```python
from build123d import *

# Parameters (mm, degrees)
SKETCH_1_W          = 1980
SKETCH_1_H          = 530
SKETCH_1_W_2        = 1920
SKETCH_1_H_2        = 470
EXTRUDE_1_DEPTH     = 30
SKETCH_2_W          = 68
SKETCH_2_H          = 30
EXTRUDE_2_DEPTH     = 68
SKETCH_3_R          = 23.5
CUT_EXTRUDE_1_DEPTH = 1125.999555555
SKETCH_4_W          = 31
SKETCH_4_H          = 470
EXTRUDE_3_DEPTH     = 30
SKETCH_5_R          = 3
CUT_EXTRUDE_2_DEPTH = 1030.528532873
SKETCH_6_R          = 3
CUT_EXTRUDE_3_DEPTH = 1030.528532873
SKETCH_7_W          = 917.525313644
SKETCH_7_H          = 30
CUT_EXTRUDE_4_DEPTH = 1125.999555555
SKETCH_8_R          = 3
CUT_EXTRUDE_5_DEPTH = 1125.999555555
SKETCH_9_R          = 3
CUT_EXTRUDE_6_DEPTH = 1028.107102497
SKETCH_10_R         = 3
CUT_EXTRUDE_7_DEPTH = 1125.999555555


with BuildPart() as part:
    # 草图1 → 凸台-拉伸1 (new body)
    with BuildSketch(Plane(origin=(0, 0, 0), x_dir=(1, 0, 0), z_dir=(0, 1, 0))):
        Rectangle(SKETCH_1_W, SKETCH_1_H)
        Rectangle(SKETCH_1_W_2, SKETCH_1_H_2, mode=Mode.SUBTRACT)
    extrude(amount=EXTRUDE_1_DEPTH)

    # 草图2 → 凸台-拉伸2 (add)
    with BuildSketch(Plane.XZ):
        with Locations((0, 250)):
            Rectangle(SKETCH_2_W, SKETCH_2_H)
        with Locations((0, -250)):
            Rectangle(SKETCH_2_W, SKETCH_2_H)
    extrude(amount=EXTRUDE_2_DEPTH)

    # 草图3 → 切除-拉伸1 (cut, through all)
    with BuildSketch(Plane.XY.offset(265)):
        with Locations((0, -30)):
            Circle(SKETCH_3_R)
    extrude(amount=-CUT_EXTRUDE_1_DEPTH, mode=Mode.SUBTRACT)

    # 草图4 → 凸台-拉伸3 (add)
    with BuildSketch(Plane(origin=(0, 30, 0), x_dir=(1, 0, 0), z_dir=(0, 1, 0))):
        with Locations((764.5, 0)):
            Rectangle(SKETCH_4_W, SKETCH_4_H)
    extrude(amount=-EXTRUDE_3_DEPTH)

    # 草图5 → 切除-拉伸2 (cut, through all)
    with BuildSketch(Plane(origin=(0, 30, 0), x_dir=(1, 0, 0), z_dir=(0, 1, 0))):
        with Locations(Location((757, 180, 0), (0, 0, 270))):
            Circle(SKETCH_5_R)
        with Locations(Location((772.5, 180, 0), (0, 0, 270))):
            Circle(SKETCH_5_R)
        with Locations(Location((757, -180, 0), (0, 0, 270))):
            Circle(SKETCH_5_R)
        with Locations(Location((772.5, -180, 0), (0, 0, 270))):
            Circle(SKETCH_5_R)
    extrude(amount=-CUT_EXTRUDE_2_DEPTH, mode=Mode.SUBTRACT)

    # 草图6 → 切除-拉伸3 (cut, symmetric)
    with BuildSketch(Plane(origin=(0, 30, 0), x_dir=(1, 0, 0), z_dir=(0, 1, 0))):
        with Locations(Location((840, -250, 0), (0, 0, 270))):
            Circle(SKETCH_6_R)
    cut_extrude_3 = extrude(amount=CUT_EXTRUDE_3_DEPTH, both=True, mode=Mode.SUBTRACT)

    # 镜向1: 切除-拉伸3 across plane
    add(cut_extrude_3.mirror(Plane.XY), mode=Mode.SUBTRACT)

    # 草图7 → 切除-拉伸4 (cut, through all)
    with BuildSketch(Plane.XY.offset(265)):
        with Locations((-608.762656822, 15)):
            Rectangle(SKETCH_7_W, SKETCH_7_H)
    extrude(amount=-CUT_EXTRUDE_4_DEPTH, mode=Mode.SUBTRACT)

    # 草图8 → 切除-拉伸5 (cut, through all)
    with BuildSketch(Plane.XY.offset(265)):
        with Locations((-100, 15)):
            Circle(SKETCH_8_R)
    extrude(amount=-CUT_EXTRUDE_5_DEPTH, mode=Mode.SUBTRACT)

    # 草图9 → 切除-拉伸6 (cut, through all)
    with BuildSketch(Plane.XZ):
        with Locations(Location((110, 250, 0), (0, 0, 270))):
            Circle(SKETCH_9_R)
        with Locations(Location((44, 250, 0), (0, 0, 270))):
            Circle(SKETCH_9_R)
    cut_extrude_6 = extrude(amount=-CUT_EXTRUDE_6_DEPTH, mode=Mode.SUBTRACT)

    # 镜向2: 切除-拉伸6 across plane
    add(cut_extrude_6.mirror(Plane.XY), mode=Mode.SUBTRACT)

    # 草图10 → 切除-拉伸7 (cut, through all)
    with BuildSketch(Plane.XY.offset(265)):
        with Locations((-135, 15)):
            Circle(SKETCH_10_R)
    extrude(amount=-CUT_EXTRUDE_7_DEPTH, mode=Mode.SUBTRACT)


solid = part.part
```
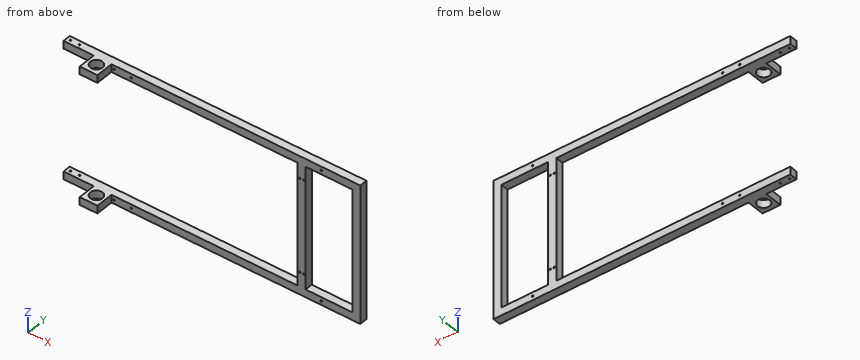
Check sheet for the modelled part. Datum: model origin and axes. Units: mm. Coordinates: 2 decimals unless noted, no trailing zeros. Loops run counter-clockwise (first coordinate to the right, second up) from the corner with the lowest first, then second, coordinate; pieces in that order, holes last.
1) Material ranges on probe 1 along X at (y, z) = (21, -180); probe 2 along X at (y, z) = (22.25, -250); probe 3 along X at (y, z) = (5.5, -127), recorded low to high.
2) Sectioned sample at C-C (y = -30). Record the boundary of the cut face in (x, z).
3) Gauge pin test, flat ends, axial feed: pin 1 (3.5 mm diameter, centred on x = 757, z = -180, fed in from -Y); pin 2 (15 mm diameter, centred on y = 9.5, z = -82, fed in from -X); pin 3 (24 mm diameter, centred on y = -35.5, z = -257.5, fed in from +X). Record the tip position at first contact, or that the pin passes through.
4) Sectioned sample at B-B (z = 77). Record the boundary of the cut face in (x, y).
5) Sectioned sample at A-A (x = 334). Record the boundary of the cut face in (y, z), and give its area (3 significant figures).
Check sheet entries:
1. probe 1: x = 749 to 754, 760 to 769.5, 775.5 to 780, 960 to 990
1. probe 2: x = -150 to 41, 47 to 107, 113 to 837, 843 to 990
1. probe 3: x = 749 to 780, 960 to 990
2. outline: (-34, -265) - (-23.5, -265) - (-23.5, -235) - (-34, -235) - close; (-34, 235) - (-23.5, 235) - (-23.5, 265) - (-34, 265) - close; (23.5, -265) - (34, -265) - (34, -235) - (23.5, -235) - close; (23.5, 235) - (34, 235) - (34, 265) - (23.5, 265) - close
3. pin 1: passes through
3. pin 2: stops at x = 749
3. pin 3: stops at x = 34
4. outline: (749, 0) - (780, 0) - (780, 30) - (749, 30) - close; (960, 0) - (990, 0) - (990, 30) - (960, 30) - close
5. outline: (0, -265) - (30, -265) - (30, -235) - (0, -235) - close; (0, 235) - (30, 235) - (30, 265) - (0, 265) - close
5. area: 1,800 mm2
